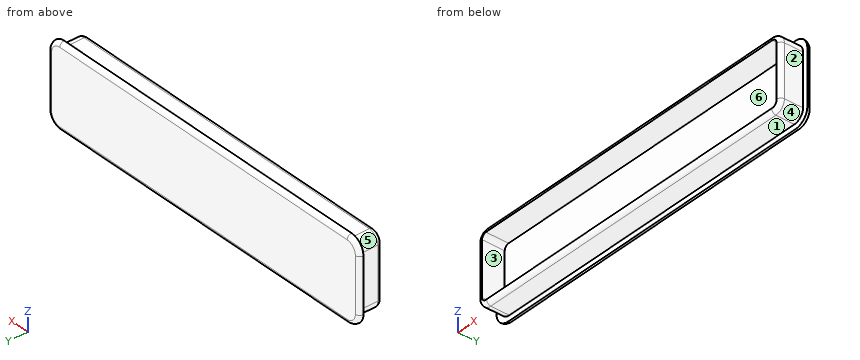
from build123d import *

# Parameters (mm, degrees)
SKETCH004_W             = 80
SKETCH004_H             = 18
PAD001_DEPTH            = 1
FILLET001_R             = 3
PAD002_DEPTH            = 5
POCKET001_DEPTH         = 5
FILLET009_R             = 0.9
FILLET010_R             = 0.9
BODY001_PLACEMENT_ANGLE = 90


with BuildPart() as part:
    # Sketch004 → Pad001 (new body)
    with BuildSketch(Plane.YZ):
        with Locations((8.97, 0.91)):
            Rectangle(SKETCH004_W, SKETCH004_H)
    extrude(amount=PAD001_DEPTH)

    # Fillet001
    fillet001_edges = [part.edges().sort_by_distance(p)[0] for p in [
        (0.5, -31.03, -8.09),
        (0.5, -31.03, 9.91),
        (0.5, 48.97, 9.91),
        (0.5, 48.97, -8.09),
    ]]
    fillet(fillet001_edges, radius=FILLET001_R)

    # Sketch005 (on Face2 of Fillet001) → Pad002 (join)
    with BuildSketch(Plane(origin=(0, 0, 0), x_dir=(0, 1, 0), z_dir=(-1, 0, 0))):
        with BuildLine():
            Line((-27.73, 6.99), (45.67, 6.99))
            ThreePointArc((47.87, 4.79), (47.225635, 6.345635), (45.67, 6.99))
            Line((47.87, 4.79), (47.87, -6.61))
            ThreePointArc((45.67, -8.81), (47.225635, -8.165635), (47.87, -6.61))
            Line((45.67, -8.81), (-27.73, -8.81))
            ThreePointArc((-29.93, -6.61), (-29.285635, -8.165635), (-27.73, -8.81))
            Line((-29.93, -6.61), (-29.93, 4.79))
            ThreePointArc((-27.73, 6.99), (-29.285635, 6.345635), (-29.93, 4.79))
        make_face()
    extrude(amount=PAD002_DEPTH)

    # Sketch006 (on Face19 of Pad002) → Pocket001 (cut)
    with BuildSketch(Plane(origin=(-5, 0, 0), x_dir=(0, 1, 0), z_dir=(-1, 0, 0))):
        with BuildLine():
            Line((-27.93, 5.99), (45.87, 5.99))
            ThreePointArc((46.87, 4.99), (46.577107, 5.697107), (45.87, 5.99))
            Line((46.87, 4.99), (46.87, -6.81))
            ThreePointArc((45.87, -7.81), (46.577107, -7.517107), (46.87, -6.81))
            Line((45.87, -7.81), (-27.93, -7.81))
            ThreePointArc((-28.93, -6.81), (-28.637107, -7.517107), (-27.93, -7.81))
            Line((-28.93, -6.81), (-28.93, 4.99))
            ThreePointArc((-27.93, 5.99), (-28.637107, 5.697107), (-28.93, 4.99))
        make_face()
    extrude(amount=-POCKET001_DEPTH, mode=Mode.SUBTRACT)

    # Fillet009
    fillet009_edges = [part.edges().sort_by_distance(p)[0] for p in [
        (1, 8.97, -8.09),
    ]]
    fillet(fillet009_edges, radius=FILLET009_R)

    # Fillet010
    fillet010_edges = [part.edges().sort_by_distance(p)[0] for p in [
        (-5, 8.97, -6.99),
    ]]
    fillet(fillet010_edges, radius=FILLET010_R)


with BuildPart() as part_1:
    # Body001 placement: moved
    add(part.part.moved(Location((9, 84.100505, 8.100505))).rotate(Axis((9, 84.100505, 8.100505), (0, 0, 1)), BODY001_PLACEMENT_ANGLE))


solid = part_1.part
The model under review builds one solid part; all positions refer to its coordinate system, in mm. Face numbers are marked on the shaded views. A direction names the side the tool comes from. Coordinates: 2 decimals unless noted, no trailing zeros. Loops run counter-clockwise (first coordinate to the right, second up) from the corner with the lowest first, then second, coordinate; pieces in that order, holes last. Notation, with made-up numbers: (-4, 43.5) -> (20, 43.5) arc R27 cw to (20, 77.5) -> close; hole circle Ø11 at (62, 71). An arc over 180 degrees is marked (long way). Use a Markdown table: item, result. Add a question column.
1. Add section A-A on y = 82.25. Write out the cut boundary in (x, z).
2. Clearance check with flat-ended pins moving along their axes: pin 1 Ø1.2 at (y, z) = (82, 9) entering from -X; pin 2 Ø2 at (x, y) = (15, 81) entering from +Z; pin 3 Ø5.5 at (x, z) = (-6, 13) entering from -Y. State where each tip first meets the part, or that it passes through.
3. Draft analysis for pull direction X (two halves, no side actions). For the marked faces 1, 2 and 3, state which applies: pulls with the +X half, pulls with the -X half, needs draft (parallel to the pull), parting line crosses it, or undercut.
4. Machinability: for the marked faces 4, 5 and 6, which of the approach directions +Z, -Z, +X, -X, +Y, -Y give a long, thin tool a straight path to every point of the face, cutting with its end or side? Answer none if there is none.
5. Add section B-B on z = 8.25. Write out the cut boundary in (x, y).
6. To check wall thickness, follow line 1 (X direction, y = 83, z = 9); line 2 (Z direction, x = 7, y = 82.75); line 3 (X direction, y = 84.25, z = 13.25). State the ranges of each line that lie inside material, in increasing order.
7. Add section C-C on x = 13.5. Write out the cut boundary in (y, z).
Returned:
| question | item | result |
|---|---|---|
| 1 | outline | (-38.87, 3.31) arc R2.2 ccw to (-36.67, 1.11) -> (36.73, 1.11) arc R2.2 ccw to (38.93, 3.31) -> (38.93, 14.71) arc R2.2 ccw to (36.73, 16.91) -> (-36.67, 16.91) arc R2.2 ccw to (-38.87, 14.71) -> close; hole (-37.87, 3.11) arc R1 ccw to (-36.87, 2.11) -> (36.93, 2.11) arc R1 ccw to (37.93, 3.11) -> (37.93, 14.91) arc R1 ccw to (36.93, 15.91) -> (-36.87, 15.91) arc R1 ccw to (-37.87, 14.91) -> close |
| 2 | pin 1 | stops at x = -38.87 |
| 2 | pin 2 | stops at z = 16.91 |
| 2 | pin 3 | stops at y = 84.1 |
| 3 | face 1 | needs draft |
| 3 | face 2 | pulls with the +X half |
| 3 | face 3 | undercut |
| 4 | face 4 | -Z, +X, -Y |
| 4 | face 5 | +Z, -X, -Y |
| 4 | face 6 | -Y |
| 5 | outline | (-39.97, 84.1) -> (-38.87, 84.1) -> (-38.87, 80) arc R0.9 ccw to (-37.97, 79.1) -> (-37.87, 79.1) -> (-37.87, 84.1) -> (37.93, 84.1) -> (37.93, 79.1) -> (38.03, 79.1) arc R0.9 ccw to (38.93, 80) -> (38.93, 84.1) -> (40.03, 84.1) -> (40.03, 84.2) arc R0.9 ccw to (39.13, 85.1) -> (-39.07, 85.1) arc R0.9 ccw to (-39.97, 84.2) -> close |
| 6 | line 1 | x = -38.87 to -37.87, 37.93 to 38.93 |
| 6 | line 2 | z = 1.11 to 2.11, 15.91 to 16.91 |
| 6 | line 3 | x = -39.97 to 40.03 |
| 7 | outline | (79.1, 2.01) arc R0.9 ccw to (80, 1.11) -> (84.1, 1.11) -> (84.1, 0.01) -> (84.2, 0.01) arc R0.9 ccw to (85.1, 0.91) -> (85.1, 17.11) arc R0.9 ccw to (84.2, 18.01) -> (84.1, 18.01) -> (84.1, 16.91) -> (80, 16.91) arc R0.9 ccw to (79.1, 16.01) -> (79.1, 15.91) -> (84.1, 15.91) -> (84.1, 2.11) -> (79.1, 2.11) -> close |
